```python
from build123d import *

# Parameters (mm, degrees)
PAD_DEPTH    = 2.2
SKETCH001_R  = 14.75
SKETCH001_W  = 2.2
SKETCH001_H  = 25.8
PAD001_DEPTH = 35.6
PAD002_DEPTH = 2.2
PAD003_DEPTH = 6.5
SKETCH004_R  = 15
PAD004_DEPTH = 9
PAD005_DEPTH = 2.2
SKETCH006_W  = 18.5
SKETCH006_H  = 29.5
PAD006_DEPTH = 6.5
SKETCH007_W  = 2.2
SKETCH007_H  = 29.5
PAD007_DEPTH = 2.2
SKETCH008_W  = 2.5
SKETCH008_H  = 6.4
PAD008_DEPTH = 0.8
SKETCH009_W  = 0.8
SKETCH009_H  = 6.4
PAD009_DEPTH = 9.5


with BuildPart() as part:
    # Sketch → Pad (new body)
    with BuildSketch(Plane.XY):
        with BuildLine():
            ThreePointArc((0, -12.9), (12.9, 0), (0, 12.9))
            Line((0, 12.9), (-17.6, 12.9))
            Line((-17.6, 12.9), (-17.6, -12.9))
            Line((0, -12.9), (-17.6, -12.9))
        make_face()
    extrude(amount=PAD_DEPTH)

    # Sketch001 → Pad001 (join)
    with BuildSketch(Plane.XY.offset(2.2)):
        Circle(SKETCH001_R)
        with Locations((-16.5, 0)):
            Rectangle(SKETCH001_W, SKETCH001_H)
    extrude(amount=PAD001_DEPTH)

    # Sketch002 → Pad002 (join)
    with BuildSketch(Plane.XY.offset(37.8)):
        with BuildLine():
            Line((-17.6, 12.9), (0, 12.9))
            ThreePointArc((0, -12.9), (12.9, 0), (0, 12.9))
            Line((-17.6, -12.9), (0, -12.9))
            Line((-17.6, 12.9), (-17.6, -12.9))
        make_face()
    extrude(amount=PAD002_DEPTH)

    # Sketch003 → Pad003 (join)
    with BuildSketch(Plane.XY.offset(40)):
        Polygon((3.5, 6.062178), (-3.5, 6.062178), (-7, 0), (-3.5, -6.062178), (3.5, -6.062178), (7, 0), align=None)
    extrude(amount=PAD003_DEPTH)

    # Sketch004 → Pad004 (join)
    with BuildSketch(Plane.XY):
        Circle(SKETCH004_R)
    extrude(amount=-PAD004_DEPTH)

    # Sketch005 → Pad005 (join)
    with BuildSketch(Plane.XY.offset(-9)):
        with BuildLine():
            Line((-15, 17), (-15, -16.999987))
            Line((-15, -16.999987), (-13.25, -16.999987))
            Line((-13.25, -13.749993), (-13.25, -16.999987))
            ThreePointArc((-10.25, -13.749993), (-11.75, -12.249993), (-13.25, -13.749993))
            Line((-10.25, -13.749993), (-10.25, -16.999987))
            Line((-10.25, -16.999987), (10.25, -16.999987))
            Line((10.25, -13.749993), (10.25, -16.999987))
            ThreePointArc((13.25, -13.749993), (11.75, -12.249993), (10.25, -13.749993))
            Line((13.25, -13.749993), (13.25, -16.999987))
            Line((13.25, -16.999987), (15, -17))
            Line((15, -17), (15, 17))
            Line((15, 17), (13.25, 17))
            Line((13.25, 13.750007), (13.25, 17))
            ThreePointArc((10.25, 13.750007), (11.75, 12.250007), (13.25, 13.750007))
            Line((10.25, 13.750007), (10.25, 17))
            Line((10.25, 17), (-10.25, 17))
            Line((-10.25, 13.750007), (-10.25, 17))
            ThreePointArc((-13.25, 13.750007), (-11.75, 12.250007), (-10.25, 13.750007))
            Line((-13.25, 13.750007), (-13.25, 17))
            Line((-13.25, 17), (-15, 17))
        make_face()
    extrude(amount=-PAD005_DEPTH)

    # Sketch006 → Pad006 (join)
    with BuildSketch(Plane.XY.offset(2.2)):
        with Locations((9.25, 0)):
            Rectangle(SKETCH006_W, SKETCH006_H)
    extrude(amount=PAD006_DEPTH)

    # Sketch007 → Pad007 (join)
    with BuildSketch(Plane.XY):
        with Locations((17.4, 0)):
            Rectangle(SKETCH007_W, SKETCH007_H)
    extrude(amount=PAD007_DEPTH)

    # Sketch008 → Pad008 (join)
    with BuildSketch(Plane.XY.offset(4)):
        with Locations((19.75, 6.95)):
            Rectangle(SKETCH008_W, SKETCH008_H)
        with Locations((19.75, -6.95)):
            Rectangle(SKETCH008_W, SKETCH008_H)
    extrude(amount=PAD008_DEPTH)

    # Sketch009 → Pad009 (join)
    with BuildSketch(Plane.XY.offset(4)):
        with Locations((20.6, 6.95)):
            Rectangle(SKETCH009_W, SKETCH009_H)
        with Locations((20.6, -6.95)):
            Rectangle(SKETCH009_W, SKETCH009_H)
    extrude(amount=PAD009_DEPTH)


solid = part.part
```
The listing builds one solid part. Answer for the finished solid, in the listing's coordinates (mm). A direction names the side the tool comes from. Coordinates: 2 decimals unless noted, no trailing zeros. Loops run counter-clockwise (first coordinate to the right, second up) from the corner with the lowest first, then second, coordinate; pieces in that order, holes last. Notation, with made-up numbers: (30, 54.5) -> (49, 54.5) arc R32 cw to (49, 93.5) -> close; hole circle Ø6 at (61.25, 57). An arc over 180 degrees is marked (long way). Return JSON: item names as keys, results as strings. Group by question number.
(1) Given pin 1 Ø5 at (x, z) = (3.5, 21.5) entering from +Y; pin 2 Ø1.8 at (y, z) = (16, -9.5) entering from +X; pin 3 Ø5 at (x, z) = (-7.5, 7) entering from -Y, each flat-ended and moving along its own axis, determine where each tip first touches the part or whether it passes through.
(2) Find the intervals of material crossed by probe 1 along Z at (x, y) = (-14.5, 12); probe 2 along X at (y, z) = (-4.5, 7); probe 3 along X at (y, z) = (-9, 11), in increasing order. Write a range as from..to.
(3) A cutting plane is placed at D-D on x = -1. Write down the section's boundary in (y, z).
(4) A cutting plane is placed at B-B on z = 34. Write down the section's boundary in (x, y), and give its area (3 significant figures).
(5) Which of the six approach directions +Z, -Z, +X, -X, +Y, -Y give full straight-line access (tool end or side, diameter ignored) to faces 5 (the flat face through (0, -6.062, 43)), 6 (the cylindrical face through (11.78, -12.25, -10.08)), 7 (the flat face through (-15, 0, 37.8)), 8 (the flat face through (20.2, -7, 9)), 9 (the flat face through (-16, -12.9, 18))?
(6) A cutting plane is placed at C-C on y = -2. Write down the section's boundary in (x, z), and give its area (3 significant figures).
(7) Determine the mould class of faces 1 (the flat face through (16.3, 0, 1)), 2 (the flat face through (9, 14.75, 5)), 3 (the flat face through (20.2, 7, 9)), 4 (the cylindrical face through (12.897, -0.284, 38.885)) for opening direction X: released by +X, released by -X, zero draft, split by the parting line, or undercut.
(8) A cutting plane is placed at A-A on z = 6. Write down the section's boundary in (x, y), and give its area (3 significant figures).
The answers:
{
 "1": {"pin 1": "stops at y = 14.72", "pin 2": "stops at x = 15", "pin 3": "stops at y = -13.88"},
 "2": {"probe 1": "z = -11.2..-9, 0..2.2, 37.8..40", "probe 2": "x = -17.6..-15.4, -14.05..18.5, 20.2..21", "probe 3": "x = -17.6..-15.4, -11.69..11.69, 20.2..21"},
 "3": {"outline": "(-17, -11.2) -> (17, -11.2) -> (17, -9) -> (14.97, -9) -> (14.97, 0) -> (12.9, 0) -> (12.9, 2.2) -> (14.72, 2.2) -> (14.72, 37.8) -> (12.9, 37.8) -> (12.9, 40) -> (6.06, 40) -> (6.06, 46.5) -> (-6.06, 46.5) -> (-6.06, 40) -> (-12.9, 40) -> (-12.9, 37.8) -> (-14.72, 37.8) -> (-14.72, 2.2) -> (-12.9, 2.2) -> (-12.9, 0) -> (-14.97, 0) -> (-14.97, -9) -> (-17, -9) -> close"},
 "4": {"outline": "(-17.6, -12.9) -> (-15.4, -12.9) -> (-15.4, 12.9) -> (-17.6, 12.9) -> close; circle Ø29.5 at (0, 0)", "area": "740 mm^2"},
 "5": {"face 5": "+Z, +X, -X, -Y", "face 6": "-Z, -Y", "face 7": "none", "face 8": "+Z, +Y, -Y", "face 9": "-X, -Y"},
 "6": {"outline": "(-17.6, 0) -> (-14.87, 0) -> (-14.87, -9) -> (-15, -9) -> (-15, -11.2) -> (15, -11.2) -> (15, -9) -> (14.87, -9) -> (14.87, 0) -> (12.74, 0) -> (12.74, 2.2) -> (16.3, 2.2) -> (16.3, 0) -> (18.5, 0) -> (18.5, 8.7) -> (14.61, 8.7) -> (14.61, 37.8) -> (12.74, 37.8) -> (12.74, 40) -> (5.85, 40) -> (5.85, 46.5) -> (-5.85, 46.5) -> (-5.85, 40) -> (-17.6, 40) -> close; hole (-15.4, 2.2) -> (-14.61, 2.2) -> (-14.61, 37.8) -> (-15.4, 37.8) -> close", "area": "1,690 mm^2"},
 "7": {"face 1": "undercut", "face 2": "zero draft", "face 3": "undercut", "face 4": "released by +X"},
 "8": {"outline": "(-17.6, -12.9) -> (-15.4, -12.9) -> (-15.4, 12.9) -> (-17.6, 12.9) -> close; (0, -14.75) -> (18.5, -14.75) -> (18.5, 14.75) -> (0, 14.75) arc R14.75 ccw to start; (20.2, -10.15) -> (21, -10.15) -> (21, -3.75) -> (20.2, -3.75) -> close; (20.2, 3.75) -> (21, 3.75) -> (21, 10.15) -> (20.2, 10.15) -> close", "area": "954 mm^2"}
}
